```python
from build123d import *

# Parameters (mm, degrees)
SKETCH1_W           = 32
SKETCH1_H           = 58.8
SKETCH1_R           = 1.45
BOSS_EXTRUDE1_DEPTH = 6
BOSS_EXTRUDE2_START = 30.2
SKETCH1_3_W         = 15.8
SKETCH1_3_H         = 58.8
SKETCH1_3_R         = 2.5
SKETCH1_3_R_2       = 1.45
BOSS_EXTRUDE2_DEPTH = 30.2


with BuildPart() as part:
    # Sketch1 → Boss-Extrude1 (new body)
    with BuildSketch(Plane.YZ):
        Rectangle(SKETCH1_W, SKETCH1_H)
        with Locations(Location((-12.5, 12.5, 0), (0, 0, 270))):
            Circle(SKETCH1_R, mode=Mode.SUBTRACT)
        with Locations(Location((12.5, 12.5, 0), (0, 0, 270))):
            Circle(SKETCH1_R, mode=Mode.SUBTRACT)
        with Locations(Location((12.5, -12.5, 0), (0, 0, 270))):
            Circle(SKETCH1_R, mode=Mode.SUBTRACT)
        with Locations(Location((-12.5, -12.5, 0), (0, 0, 270))):
            Circle(SKETCH1_R, mode=Mode.SUBTRACT)
    extrude(amount=-BOSS_EXTRUDE1_DEPTH)

    # Sketch1_3 → Boss-Extrude2 (add)
    # profile 1 of 3: a face of its own
    with BuildSketch(Plane.YZ.offset(BOSS_EXTRUDE2_START)):
        with Locations((8.1, 0)):
            Rectangle(SKETCH1_3_W, SKETCH1_3_H)
        with Locations((12.5, -12.5)):
            Circle(SKETCH1_3_R, mode=Mode.SUBTRACT)
        with Locations((12.5, 12.5)):
            Circle(SKETCH1_3_R, mode=Mode.SUBTRACT)
    # profile 2 of 3: a face of its own
    with BuildSketch(Plane.YZ.offset(BOSS_EXTRUDE2_START)):
        with Locations((12.5, 12.5)):
            Circle(SKETCH1_3_R)
        with Locations(Location((12.5, 12.5, 0), (0, 0, 270))):
            Circle(SKETCH1_3_R_2, mode=Mode.SUBTRACT)
    # profile 3 of 3: a face of its own
    with BuildSketch(Plane.YZ.offset(BOSS_EXTRUDE2_START)):
        with Locations((12.5, -12.5)):
            Circle(SKETCH1_3_R)
        with Locations(Location((12.5, -12.5, 0), (0, 0, 270))):
            Circle(SKETCH1_3_R_2, mode=Mode.SUBTRACT)
    extrude(amount=-BOSS_EXTRUDE2_DEPTH)


solid = part.part
```
Input: part model. Units: mm. Frame: model coordinates. A direction names the side the tool comes from. Give positions to 0.01 mm unless a question says otherwise; leave off trailing zeros. Order: outer loops, then holes, each group sorted by start corner. A loop starts at its lowest first (then second) coordinate and runs counter-clockwise, first axis right, second up.
1. Section A-A on z = 12.5. Return the cut outline in (x, y), and give its area (3 significant figures).
Derived:
outline: (-6, -16) - (0, -16) - (0, -13.95) - (-6, -13.95) - close; (-6, -11.05) - (0, -11.05) - (0, 0.2) - (30.2, 0.2) - (30.2, 11.05) - (-6, 11.05) - close; (-6, 13.95) - (30.2, 13.95) - (30.2, 16) - (-6, 16) - close
area: 547 mm2
2. Section B-B on y = -12.5. Return the cut outline in (x, z), and give its area (3 significant figures).
Derived:
outline: (-6, -29.4) - (0, -29.4) - (0, -13.95) - (-6, -13.95) - close; (-6, -11.05) - (0, -11.05) - (0, 11.05) - (-6, 11.05) - close; (-6, 13.95) - (0, 13.95) - (0, 29.4) - (-6, 29.4) - close
area: 318 mm2
3. Reachability of faces 1 (the flat face through (0, -8, 0)), 2 (the cylindrical face through (-2.96, -13.38, -11.35)) from +Z, -Z, +X, -X, +Y, -Y: full face, straight path, thin tool, end or side. Return the list, or none.
Derived:
face 1: +Z, -Z, +X, -Y
face 2: +X, -X
4. Section C-C on x = 18. Return the cut outline in (y, z), and give its area (3 significant figures).
Derived:
outline: (0.2, -29.4) - (16, -29.4) - (16, 29.4) - (0.2, 29.4) - close; hole circle Ø2.9 at (12.5, -12.5); hole circle Ø2.9 at (12.5, 12.5)
area: 916 mm2
5. Section D-D on z = -18.5. Return the cut outline in (x, y), and give its area (3 significant figures).
Derived:
outline: (-6, -16) - (0, -16) - (0, 0.2) - (30.2, 0.2) - (30.2, 16) - (-6, 16) - close
area: 669 mm2
6. Mould query, pull axis Z, two halves, no side actions, for faces 3 (the flat face through (12, 7, -29.4)), 4 (the flat face through (12, 16, 0)), 5 (the cylindrical face through (12.35, 11.62, 13.65)). Classes: released by +Z, released by -Z, zero draft, split by the parting line, or undercut.
Derived:
face 3: released by -Z
face 4: zero draft
face 5: undercut
7. Pin query (flat end, axial travel): pin 1 (10 mm diameter, centred on x = 15.5, z = 10.5, fed in from -Y); pin 2 (8 mm diameter, centred on y = -5, z = -6.5, fed in from +X). Return the tip coordinate at first contact, or that it passes through.
Derived:
pin 1: stops at y = 0.2
pin 2: stops at x = 0
8. Material intervals for L1, parallel to Z at x = 3, y = 12; L2, parallel to Y at x = 6.5, z = -12.5; L3, parallel to X at y = -9.5, z = 22, sorted ascending.
Derived:
L1: z = -29.4 to -13.86, -11.14 to 11.14, 13.86 to 29.4
L2: y = 0.2 to 11.05, 13.95 to 16
L3: x = -6 to 0
